Part model, mm, in its own coordinate system. Face numbers are marked on the shaded views. Coordinates: 2 decimals unless noted, no trailing zeros. Order: outer loops, then holes, each group sorted by start corner. A loop starts at its lowest first (then second) coordinate and runs counter-clockwise, first axis right, second up.
1) Pin check, flat tips, straight feed: pin 1 Ø4.5 at (x, y) = (17, -10.5) entering from +Z; pin 2 Ø1.5 at (x, z) = (66, 9.5) entering from +Y; pin 3 Ø3 at (x, z) = (17, 2) entering from +Y; pin 4 Ø0.6 at (x, y) = (47.5, -28.5) entering from +Z. Stop position of each tip, or through.
2) Cut at A-A (x = 57). List the corners of the cut face in (y, z).
3) Cut at C-C (z = 9.5). List the corners of the cut face in (x, y).
4) Mould opens along X. For the marked faces 1 and 2 say: +X half, -X half, draft (parallel to the pull), parting line (faces both ways), or undercut.
5) Cut at B-B (y = -29). List the corners of the cut face in (x, z).
6) Cut at D-D (y = -22). List the corners of the cut face in (x, z).
7) Wall check: L1, parallel to Y at x = 69, z = 49.75; L2, parallel to X at y = -39, z = 33; L3, parallel to X at y = -10, z = 52. Give the ranges that are in metal, low to high.
```python
from build123d import *

# Parameters (mm, degrees)
F1_DEPTH  = 4
F2_W      = 2
F2_H      = 7.5
F3_DEPTH  = 1.7
F5_DEPTH  = 62.5
F4_R      = 3
F7_W      = 74
F7_H      = 6
F8_DEPTH  = 4
F9_R      = 1.9
F10_R     = 1.9
F11_DEPTH = 25


with BuildPart() as f1:
    # F0 (on Top) → F1 (new body)
    with BuildSketch(Plane.XY):
        with BuildLine():
            Line((6, 0), (80, 0))
            Line((80, 0), (80, -24))
            Line((80, -24), (80, -34))
            Line((80, -34), (80, -39))
            ThreePointArc((80, -39), (83, -42), (86, -39))
            Line((86, -39), (86, 15))
            ThreePointArc((86, 15), (83, 18), (80, 15))
            Line((80, 15), (80, 10))
            Line((80, 10), (50, 10))
            Line((50, 10), (50, 2.5))
            Line((50, 2.5), (38.5, 2.5))
            Line((38.5, 2.5), (38.5, 10))
            Line((38.5, 10), (20.5, 10))
            Line((20.5, 10), (20.5, 2.5))
            Line((20.5, 2.5), (9, 2.5))
            Line((9, 2.5), (9, 10))
            Line((9, 10), (6, 10))
            Line((6, 10), (6, 15))
            ThreePointArc((6, 15), (3, 18), (0, 15))
            Line((0, 15), (0, -39))
            ThreePointArc((0, -39), (3, -42), (6, -39))
            Line((6, -39), (6, -34))
            Line((6, -34), (6, -24))
            Line((6, -24), (6, 0))
        make_face()
        Polygon((80, -34), (80, -24), (50, -24), (50, -31.5), (38.5, -31.5), (38.5, -24), (20.5, -24), (20.5, -31.5), (9, -31.5), (9, -24), (6, -24), (6, -34), align=None)
    extrude(amount=F1_DEPTH)

    # F2 (on Top) → F3 (join)
    with BuildSketch(Plane.XY):
        with Locations((12, 6.25)):
            Rectangle(F2_W, F2_H)
        with Locations((17.5, 6.25)):
            Rectangle(F2_W, F2_H)
        with Locations((41.5, 6.25)):
            Rectangle(F2_W, F2_H)
        with Locations((47, 6.25)):
            Rectangle(F2_W, F2_H)
        with Locations((12, -27.75)):
            Rectangle(F2_W, F2_H)
        with Locations((17.5, -27.75)):
            Rectangle(F2_W, F2_H)
        with Locations((41.5, -27.75)):
            Rectangle(F2_W, F2_H)
        with Locations((47, -27.75)):
            Rectangle(F2_W, F2_H)
    extrude(amount=F3_DEPTH)

    # F4 (on face) → F5 (join)
    with BuildSketch(Plane.XY.offset(4)):
        with BuildLine():
            ThreePointArc((0, 15), (3, 12), (6, 15))
            ThreePointArc((6, 15), (3, 18), (0, 15))
        make_face()
        with BuildLine():
            ThreePointArc((6, -39), (3, -36), (0, -39))
            ThreePointArc((0, -39), (3, -42), (6, -39))
        make_face()
        with BuildLine():
            ThreePointArc((86, -39), (83, -36), (80, -39))
            ThreePointArc((80, -39), (83, -42), (86, -39))
        make_face()
        with BuildLine():
            ThreePointArc((80, 15), (83, 12), (86, 15))
            ThreePointArc((86, 15), (83, 18), (80, 15))
        make_face()
    extrude(amount=F5_DEPTH)



with BuildPart() as f5:
    # F4 (on face) → F5, piece 2 (new body)
    with BuildSketch(Plane.XY.offset(4)):
        with Locations((17, -10.5)):
            Circle(F4_R)
    extrude(amount=F5_DEPTH)


with BuildPart() as f5b:
    # F4 (on face) → F5, piece 3 (new body)
    with BuildSketch(Plane.XY.offset(4)):
        with Locations((69, -10.5)):
            Circle(F4_R)
    extrude(amount=F5_DEPTH)


with BuildPart() as f1_1:
    add(f1.part)

    add(f5.part)  # F8 merges F5

    add(f5b.part)  # F8 merges F5b
    # F7 (on face) → F8 (join)
    with BuildSketch(Plane(origin=(0, 0, 0), x_dir=(1, 0, 0), z_dir=(0, 0, -1))):
        with Locations((43, 10.5)):
            Rectangle(F7_W, F7_H)
    extrude(amount=-F8_DEPTH)

    # F9 (on face) + F10 (on face) → F11 (cut)
    with BuildSketch(Plane.XY.offset(66.5)):
        with Locations((17, -10.5)):
            Circle(F9_R)
    with BuildSketch(Plane.XY.offset(66.5)):
        with Locations((69, -10.5)):
            Circle(F10_R)
    extrude(amount=-F11_DEPTH, mode=Mode.SUBTRACT)


solid = f1_1.part
```
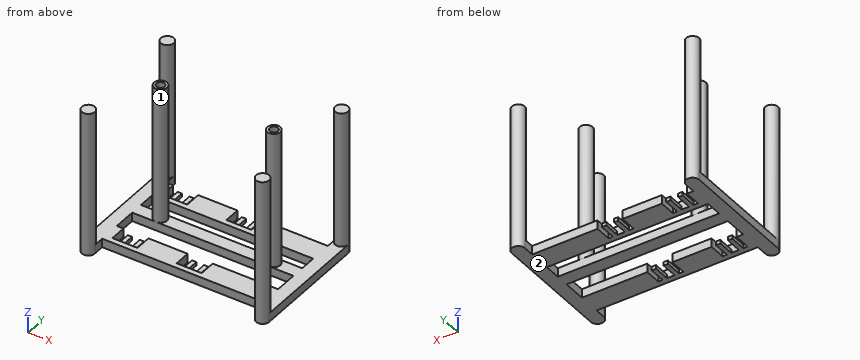
Geometry check:
1. pin 1: stops at z = 66.5
1. pin 2: stops at y = -8.52
1. pin 3: stops at y = 10
1. pin 4: stops at z = 1.7
2. outline: (-34, 0) - (-24, 0) - (-24, 4) - (-34, 4) - close; (-13.5, 0) - (-7.5, 0) - (-7.5, 4) - (-13.5, 4) - close; (0, 0) - (10, 0) - (10, 4) - (0, 4) - close
3. outline: circle Ø6 at (3, -39); circle Ø6 at (3, 15); circle Ø6 at (17, -10.5); circle Ø6 at (69, -10.5); circle Ø6 at (83, -39); circle Ø6 at (83, 15)
4. face 1: undercut
4. face 2: draft
5. outline: (0, 0) - (9, 0) - (9, 4) - (0, 4) - close; (11, 0) - (13, 0) - (13, 1.7) - (11, 1.7) - close; (16.5, 0) - (18.5, 0) - (18.5, 1.7) - (16.5, 1.7) - close; (20.5, 0) - (38.5, 0) - (38.5, 4) - (20.5, 4) - close; (40.5, 0) - (42.5, 0) - (42.5, 1.7) - (40.5, 1.7) - close; (46, 0) - (48, 0) - (48, 1.7) - (46, 1.7) - close; (50, 0) - (86, 0) - (86, 4) - (50, 4) - close
6. outline: (0, 0) - (6, 0) - (6, 4) - (0, 4) - close; (80, 0) - (86, 0) - (86, 4) - (80, 4) - close
7. L1: y = -13.5 to -12.4, -8.6 to -7.5
7. L2: x = 0 to 6, 80 to 86
7. L3: x = 14.04 to 15.17, 18.83 to 19.96, 66.04 to 67.17, 70.83 to 71.96
